from build123d import *

# Parameters (mm, degrees)
BOSS_EXTRUDE1_DEPTH = 35
BOSS_EXTRUDE2_DEPTH = 3.5
BOSS_EXTRUDE3_DEPTH = 2
CUT_EXTRUDE2_DEPTH  = 0.5
FILLET1_R           = 0.8
SKETCH5_R           = 1.75
BOSS_EXTRUDE4_DEPTH = 5
FILLET2_R           = 0.8
SKETCH6_R           = 2.5
CUT_EXTRUDE4_DEPTH  = 128.140994275


with BuildPart() as part:
    # Sketch1 → Boss-Extrude1 (new body)
    with BuildSketch(Plane.XY):
        with BuildLine():
            ThreePointArc((32.5, 3.5), (60.216385975, -15.019497029), (53.713203436, -47.713203436))
            Line((53.713203436, -47.713203436), (51.238329701, -45.238329701))
            ThreePointArc((51.238329701, -45.238329701), (56.982807612, -16.358889042), (32.5, 0))
            Line((32.5, 0), (-32.5, 0))
            ThreePointArc((-32.5, 0), (-56.982807612, -16.358889042), (-51.238329701, -45.238329701))
            Line((-51.238329701, -45.238329701), (-53.713203436, -47.713203436))
            ThreePointArc((-53.713203436, -47.713203436), (-60.216385975, -15.019497029), (-32.5, 3.5))
            Line((-32.5, 3.5), (32.5, 3.5))
        make_face()
    extrude(amount=BOSS_EXTRUDE1_DEPTH)

    # Sketch2 → Boss-Extrude2 (add)
    with BuildSketch(Plane(origin=(-50.713203436, -50.713203436, 0), x_dir=(0, 0, 1), z_dir=(-0.7071067811865488, -0.7071067811865464, 0))):
        with BuildLine():
            Line((35, 4.242640687), (0, 4.242640687))
            ThreePointArc((0, 4.242640687), (17.5, -13.257359313), (35, 4.242640687))
        make_face()
    boss_extrude2 = extrude(amount=-BOSS_EXTRUDE2_DEPTH)

    # Mirror1: Boss-Extrude2 across plane
    add(boss_extrude2.mirror(Plane(origin=(0, 0, 0), x_dir=(0, 0, 1), z_dir=(1, 0, 0))))

    # Sketch3 → Boss-Extrude3 (add)
    with BuildSketch(Plane(origin=(-50.713203436, -50.713203436, 0), x_dir=(0, 0, 1), z_dir=(-0.7071067811865487, -0.7071067811865465, 0))):
        Polygon((17.502560815, -0.889154327), (9.378087293, -12.279246125), (17.502560815, -21.961616632), (25.627034337, -12.279246125), align=None)
    extrude(amount=BOSS_EXTRUDE3_DEPTH)

    # Sketch4 → Cut-Extrude2 (cut)
    with BuildSketch(Plane(origin=(-52.127416998, -52.127416998, 0), x_dir=(0, 0, 1), z_dir=(-0.7071067811865486, -0.7071067811865465, 0))):
        Polygon((11.432409465, -11.094265864), (17.402560815, -9.038577899), (17.402560815, -2.724422361), align=None)
        Polygon((17.602560815, -9.038577899), (23.572712164, -11.094265864), (17.602560815, -2.724422361), align=None)
        Polygon((17.402560815, -9.250102035), (11.40902714, -11.31384118), (17.402560815, -14.36769912), align=None)
        Polygon((17.602560815, -14.36769912), (23.59609449, -11.31384118), (17.602560815, -9.250102035), align=None)
        Polygon((17.402560815, -15.714490605), (11.524861695, -12.719653319), (17.402560815, -19.724422361), align=None)
        Polygon((17.602560815, -19.724422361), (23.480259935, -12.719653319), (17.602560815, -15.714490605), align=None)
    extrude(amount=-CUT_EXTRUDE2_DEPTH, mode=Mode.SUBTRACT)

    # Fillet1
    fillet1_edges = [part.edges().sort_by_distance(p)[0] for p in [
        (-42.737572014, -60.103048419, 25.627034337),
        (-50.791583162, -52.049037271, 17.502560815),
        (-42.737572014, -60.103048419, 9.378087293),
        (-35.89110217, -66.949518263, 17.502560815),
    ]]
    fillet(fillet1_edges, radius=FILLET1_R)

    # Sketch5 → Boss-Extrude4 (add)
    with BuildSketch(Plane(origin=(-48.238329701, -48.238329701, 0), x_dir=(0, 0, -1), z_dir=(0.7071067811865487, 0.7071067811865465, 0))):
        with Locations(Location((-17.5, -4.757359313, 0), (0, 0, 90))):
            Circle(SKETCH5_R)
    extrude(amount=BOSS_EXTRUDE4_DEPTH)

    # Fillet2
    fillet2_edges = [part.edges().sort_by_distance(p)[0] for p in [
        (-40.101397898, -49.304193693, 17.5),
    ]]
    fillet(fillet2_edges, radius=FILLET2_R)

    # Sketch6 → Cut-Extrude4 (cut, through all)
    with BuildSketch(Plane(origin=(48.238329701, -48.238329701, 0), x_dir=(0, 0, 1), z_dir=(-0.7071067811865487, 0.7071067811865465, 0))):
        with Locations((17.5, 4.242640687)):
            Circle(SKETCH6_R)
    extrude(amount=-CUT_EXTRUDE4_DEPTH, mode=Mode.SUBTRACT)


solid = part.part
Read the model definition and answer for the solid it produces. Units are mm, in the model's axes. A direction names the side the tool comes from. Round coordinates to 2 decimals unless told otherwise and drop trailing zeros. Write each loop counter-clockwise with the first axis right and the second up, starting at its lowest first coordinate (ties: lowest second). Pieces come first, ordered by that corner, then holes. Notation, with made-up numbers: M 29.5,89.25 L 67.5,89.25 A25 ccw 67.5,125.25 Z; hole C 16,2.25 d6. An arc over 180 degrees is marked long. Use a Markdown table: item, result.
1) For a pull along X with two mould halves and no side action, classify faces 1 (the cylindrical face through (60.02, -14.56, 17.26)), 2 (the cylindrical face through (57.147, -16.764, 17.255)), 3 (the cylindrical face through (-60.402, -15.478, 17.255)) as pulls with the +X half, pulls with the -X half, needs draft (parallel to the pull), parting line crosses it, or undercut.
Answers follow:
| item | result |
|---|---|
| face 1 | pulls with the +X half |
| face 2 | undercut |
| face 3 | pulls with the -X half |
2) The part is cut by section C-C (x = -5). Write down the section's boundary in (y, z), plus the area to 4 significant figures.
Answers follow:
| item | result |
|---|---|
| outline | M 0,0 L 3.5,0 L 3.5,35 L 0,35 Z |
| area | 122.5 mm2 |
3) The part is cut by section D-D (y = -2). Write down the section's boundary in (x, z).
Answers follow:
| item | result |
|---|---|
| outline | M -49.81,0 L -42.6,0 L -42.6,35 L -49.81,35 Z; M 42.6,0 L 49.81,0 L 49.81,35 L 42.6,35 Z |
4) A tool of negligible diameter and unlimited length cuts with its end or side. For faces 4 (the cylindrical face through (52.5, -46.4, 15)), 5 (the flat face through (48.988, -52.439, 17.255)), 6 (the flat face through (-46.66, -56.161, 13.344)), 7 (the cylindrical face through (-56.812, -15.956, 17.255)), from which of +Z, -Z, +X, -X, +Y, -Y can it reach the whole face along a straight path? Write none if from no direction.
Answers follow:
| item | result |
|---|---|
| face 4 | none |
| face 5 | +Z, -Z, +X, -Y |
| face 6 | -Z, -X |
| face 7 | +Z, -Z |
5) The part is cut by section B-B (z = 5.5). Write down the section's boundary in (x, y).
Answers follow:
| item | result |
|---|---|
| outline | M -53.71,-47.71 L -44.71,-56.72 L -42.23,-54.25 L -51.24,-45.24 A26.5 cw -32.5,0 L 32.5,0 A26.5 cw 51.24,-45.24 L 42.23,-54.25 L 44.71,-56.72 L 53.71,-47.71 A30 ccw 32.5,3.5 L -32.5,3.5 A30 ccw Z |
6) The part is cut by section A-A (y = -35). Write down the section's boundary in (x, z), plus the area to 3 significant figures.
Answers follow:
| item | result |
|---|---|
| outline | M -61.27,0 L -57.6,0 L -57.6,35 L -61.27,35 Z; M 57.6,0 L 61.27,0 L 61.27,35 L 57.6,35 Z |
| area | 257 mm2 |
7) Straight lines are drawn through the part: line 1 along Y through (x, z) = (-50, 17.5); line 2 along Y through (x, z) = (-23.5, 15); line 3 along Y through (x, z) = (-57, 16.5). For each, find the intervals that lie inside material, in ascending order. Write a range as [from, to].
Answers follow:
| item | result |
|---|---|
| line 1 | y = [-54.25, -52.07], [-51.43, -46.48], [-6.6, -2.13] |
| line 2 | y = [0, 3.5] |
| line 3 | y = [-43.81, -36.6], [-16.4, -9.19] |
8) Flat-ended cylindrical pins translate along their axes: pin 1 (4 mm diameter, centred on x = -12, z = 20.5, fed in from -Y); pin 2 (2.5 mm diameter, centred on x = -39, y = -65, fed in from -Z); pin 3 (3 mm diameter, centred on x = -43.5, y = -59.5, fed in from -Z). Find the tip coordinate at first contact, or state that the pin passes through.
Answers follow:
| item | result |
|---|---|
| pin 1 | stops at y = 0 |
| pin 2 | stops at z = 13.45 |
| pin 3 | stops at z = 7.78 |
